```python
from build123d import *

# Parameters (mm, degrees)
F0_W     = 19.05
F0_H     = 38.1
F1_DEPTH = 35.56
F2_W     = 31.75
F2_H     = 12.7
F3_DEPTH = 25.4
F5_DEPTH = 35.561
F6_R     = 3.175
F7_DEPTH = 6.35


with BuildPart() as f1:
    # F0 (on Top) → F1 (new body)
    with BuildSketch(Plane.XY):
        with Locations((9.525, 19.05)):
            Rectangle(F0_W, F0_H)
    extrude(amount=-F1_DEPTH)

    # F2 (on face) → F3 (cut)
    with BuildSketch(Plane(origin=(0, 0, 0), x_dir=(0, -1, 0), z_dir=(-1, 0, 0))):
        with Locations((-22.225, -17.78)):
            Rectangle(F2_W, F2_H)
    extrude(amount=-F3_DEPTH, mode=Mode.SUBTRACT)

    # F4 (on face) → F5 (cut, through all)
    with BuildSketch(Plane.XY):
        with BuildLine():
            ThreePointArc((12.7, 25.397724), (7.279936, 27.642788), (9.525, 22.222724))
            ThreePointArc((9.525, 22.222724), (11.770064, 23.15266), (12.7, 25.397724))
        make_face()
    extrude(amount=-F5_DEPTH, mode=Mode.SUBTRACT)

    # F6 (on face) → F7 (cut)
    with BuildSketch(Plane.XZ):
        with Locations((6.35, -30.7848)):
            Circle(F6_R)
        with Locations((6.35, -4.7752)):
            Circle(F6_R)
    extrude(amount=-F7_DEPTH, mode=Mode.SUBTRACT)


solid = f1.part
```
The listing builds one solid part. Answer for the finished solid, in the listing's coordinates (mm). A direction names the side the tool comes from. Coordinates: 2 decimals unless noted, no trailing zeros. Loops run counter-clockwise (first coordinate to the right, second up) from the corner with the lowest first, then second, coordinate; pieces in that order, holes last. Notation, with made-up numbers: (47, 70.25) -> (78, 70.25) arc R23 cw to (78, 79.25) -> close; hole circle Ø10 at (7, 85). An arc over 180 degrees is marked (long way). Return JSON: item names as keys, results as strings. Group by question number.
(1) Determine the mould class of faces 1 (the flat face through (6, 6.35, -5)), 2 (the flat face through (9, 6.35, -18)), 3 (the flat face through (19.05, 19, -10)), 4 (the flat face through (9, 19, -35.56)) for opening direction Z: released by +Z, released by -Z, zero draft, split by the parting line, or undercut.
(2) A cutting plane is placed at B-B on x = 10.25. Write down the section's boundary in (y, z).
(3) Find the intervals of material crossed by probe 1 along Z at (x, y) = (6.35, 3.75); probe 2 along Z at (x, y) = (1.25, 9.5); probe 3 along X at (y, z) = (3, -31), in increasing order. Write a range as from..to.
(4) A cutting plane is placed at A-A on y = 19. Write down the section's boundary in (x, z).
(5) Which of the six approach directions +Z, -Z, +X, -X, +Y, -Y give full straight-line access (tool end or side, diameter ignored) to faces 5 (the flat face through (12, 22, -11.43)), 6 (the cylindrical face through (5.937, 3.131, -27.637)), 7 (the flat face through (9, 38.1, -30))?
(6) A cutting plane is placed at D-D on z = -20. Write down the section's boundary in (x, y), and give its area (3 significant figures).
(7) Given pin 1 Ø1.9 at (x, z) = (6, -30.5) entering from -Y; pin 2 Ø10 at (x, z) = (8.5, -17) entering from +Y, each flat-ended and moving along its own axis, determine where each tip first touches the part or whether it passes through.
(8) A cutting plane is placed at C-C on z = -9. Write down the section's boundary in (x, y) (3 decimals).
The answers:
{
 "1": {"face 1": "undercut", "face 2": "undercut", "face 3": "zero draft", "face 4": "released by -Z"},
 "2": {"outline": "(0, -35.56) -> (22.31, -35.56) -> (22.31, -24.13) -> (6.35, -24.13) -> (6.35, -11.43) -> (22.31, -11.43) -> (22.31, 0) -> (0, 0) -> close; (28.49, -35.56) -> (38.1, -35.56) -> (38.1, -24.13) -> (28.49, -24.13) -> close; (28.49, -11.43) -> (38.1, -11.43) -> (38.1, 0) -> (28.49, 0) -> close"},
 "3": {"probe 1": "z = -35.56..-33.96, -27.61..-7.95, -1.6..0", "probe 2": "z = -35.56..-24.13, -11.43..0", "probe 3": "x = 0..3.18, 9.52..19.05"},
 "4": {"outline": "(0, -35.56) -> (19.05, -35.56) -> (19.05, -24.13) -> (0, -24.13) -> close; (0, -11.43) -> (19.05, -11.43) -> (19.05, 0) -> (0, 0) -> close"},
 "5": {"face 5": "+X, -X, +Y", "face 6": "-Y", "face 7": "+Z, -Z, +X, -X, +Y"},
 "6": {"outline": "(0, 0) -> (19.05, 0) -> (19.05, 6.35) -> (0, 6.35) -> close", "area": "121 mm^2"},
 "7": {"pin 1": "stops at y = 6.35", "pin 2": "stops at y = 6.35"},
 "8": {"outline": "(0, 0) -> (19.05, 0) -> (19.05, 38.1) -> (0, 38.1) -> close; hole circle Ø6.35 at (9.525, 25.398)"}
}
